Input: dimensioned drawing with shaded views. Units: mm. Origin: part minimum x, y, z. A direction names the side the tool comes from. Round coordinates to 2 decimals unless told otherwise and drop trailing zeros. Write each loop counter-clockwise with the first axis right and the second up, starting at its lowest first coordinate (ties: lowest second). Pieces come first, ordered by that corner, then holes. Notation, with made-up numbers: (86, 22.25) -> (105, 22.25) arc R29 cw to (105, 57.25) -> close; hole circle Ø2 at (54.25, 46.25). An arc over 180 degrees is marked (long way). Return JSON: item names as keys, results as strings. Group by question number.
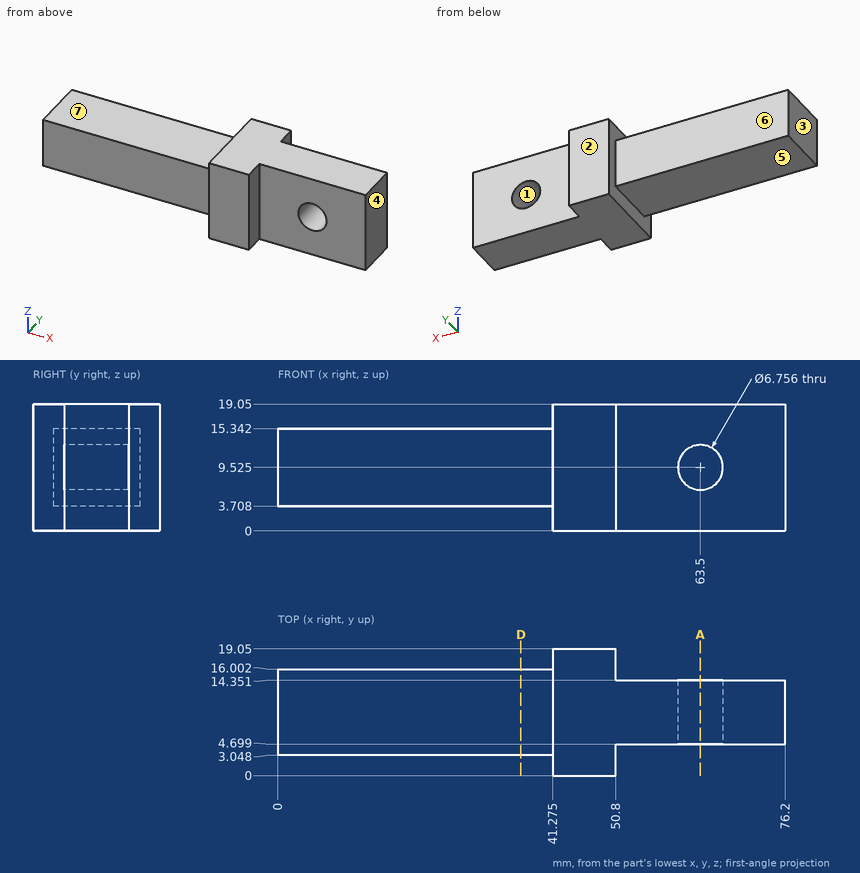
Item 1: Material intervals for probe 1 along Z at (x, y) = (63.5, 11.25); probe 2 along X at (y, z) = (16.25, 3.5) (1 decimal); probe 3 along X at (y, z) = (15, 15), sorted ascending.
Item 2: Cut plane A-A on x = 63.5. Output: boundary loops of the cut face in (y, z), and give its area (3 significant figures).
Item 3: Pull-direction query (X, two-part tool) for the marked faces 1, 2, 3 and 4; classes: +X half, -X half, draft (parallel to the pull), parting line (faces both ways), or undercut.
Item 4: First-contact query: pin 1 Ø6 at (x, z) = (29, 3.5) entering from -Y; pin 2 Ø10 at (x, y) = (34.5, 10) entering from +Z; pin 3 Ø2 at (x, y) = (10.5, 8) entering from -Z. Flat tips, straight axial feed; report the tip coordinate or a pass-through.
Item 5: Set-up query: the marked faces 5, 6 and 7. Return all of +Z, -Z, +X, -X, +Y, -Y with unobstructed straight access to the full face (end or side cutting, diameter ignored); none if empty.
Item 6: Cut plane D-D on x = 36.5. Output: boundary loops of the cut face in (y, z), and give its area (3 significant figures).
Here are the results:
{
 "1": {"probe 1": "z = 0 to 6.15, 12.9 to 19.05", "probe 2": "x = 41.3 to 50.8", "probe 3": "x = 0 to 50.8"},
 "2": {"outline": "(4.7, 0) -> (14.35, 0) -> (14.35, 6.15) -> (4.7, 6.15) -> close; (4.7, 12.9) -> (14.35, 12.9) -> (14.35, 19.05) -> (4.7, 19.05) -> close", "area": "119 mm^2"},
 "3": {"face 1": "undercut", "face 2": "draft", "face 3": "-X half", "face 4": "+X half"},
 "4": {"pin 1": "stops at y = 3.05", "pin 2": "stops at z = 15.34", "pin 3": "stops at z = 3.71"},
 "5": {"face 5": "-Z, -X, +Y, -Y", "face 6": "+Z, -Z, -X, +Y", "face 7": "+Z, -X, +Y, -Y"},
 "6": {"outline": "(3.05, 3.71) -> (16, 3.71) -> (16, 15.34) -> (3.05, 15.34) -> close", "area": "151 mm^2"}
}
